Here's how the part is built. I have some questions about the finished solid (model axes, mm). Face numbers are marked on the shaded views. A direction names the side the tool comes from. Coordinates: 2 decimals unless noted, no trailing zeros. Write each loop counter-clockwise with the first axis right and the second up, starting at its lowest first coordinate (ties: lowest second). Pieces come first, ordered by that corner, then holes.
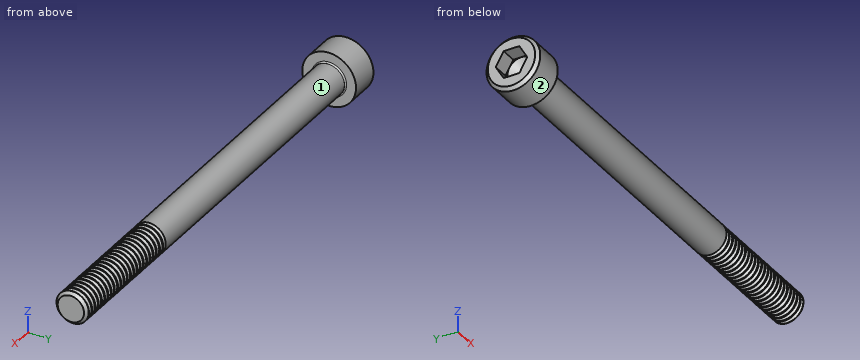
```python
from build123d import *

# Parameters (mm, degrees)
FILLET1_R       = 0.25
HEX_2_DEPTH     = 3
THDSCHPAT_COUNT = 24
THDSCHPAT_PITCH = 1


with BuildPart() as part:
    # BodySke → Base-Revolve (revolve)
    with BuildSketch(Plane.XY):
        Polygon((0, 0), (0, 4.4), (0.6, 5), (6, 5), (6, 3), (85.4455, 3), (86, 2.4455), (86, 0), align=None)
    revolve(axis=Axis((-31.75, 0, 0), (1, 0, 0)))

    # Fillet1
    fillet1_edges = [part.edges().sort_by_distance(p)[0] for p in [
        (6, -3, 0),
    ]]
    fillet(fillet1_edges, radius=FILLET1_R)

    # Sketch2 → Hex-PreBroach (revolve, cut)
    with BuildSketch(Plane.XY):
        Polygon((0, 2.542), (3, 2.542), (4.467624384, 0), (0, 0), align=None)
    revolve(axis=Axis((0, 0, 0), (1, 0, 0)), mode=Mode.SUBTRACT)

    # Sketch3 → Hex 2 (cut)
    with BuildSketch(Plane(origin=(0, 0, 0), x_dir=(0, 0.5, 0.866025404), z_dir=(-1, 0, 0))):
        Polygon((1.467624384, 2.542), (-1.467624384, 2.542), (-2.935248769, 0), (-1.467624384, -2.542), (1.467624384, -2.542), (2.935248769, 0), align=None)
    extrude(amount=-HEX_2_DEPTH, mode=Mode.SUBTRACT)

    # ThdSchSke → ThreadSchematic (revolve, cut)
    with BuildSketch(Plane.XY):
        Polygon((62, -2.4455), (61.61173492, -3), (61.61173492, -3.75), (62.38826508, -3.75), (62.38826508, -3), align=None)
    threadschematic = revolve(axis=Axis((-3.175, 0, 0), (1, 0, 0)), mode=Mode.SUBTRACT)

    # ThdSchPat: ThreadSchematic ×24
    with Locations(*[(i * THDSCHPAT_PITCH, 0, 0) for i in range(1, THDSCHPAT_COUNT)]):
        add(threadschematic, mode=Mode.SUBTRACT)


solid = part.part
```
1) Will these pins go through, and if not, where does the flat tip stop? pin 1 (5 mm diameter, centred on x = 43.5, y = 4, fed in from -Z); pin 2 (2 mm diameter, centred on x = 24, y = 0, fed in from +Z); pin 3 (1.5 mm diameter, centred on x = 74, z = -2.5, fed in from -Y).
Values follow:
pin 1: stops at z = -2.6
pin 2: stops at z = 3
pin 3: stops at y = -2.36
2) Imagine slicing it at A-A on x = 24.5. Please give me the cut outline in (y, z).
Values follow:
outline: circle Ø6 at (0, 0)
3) I need wall thicknesses on probe 1 along Z at (x, y) = (26.5, -0.25); probe 2 along Y at (x, z) = (5, -4); probe 3 along X at (y, z) = (1, 3.5). Which ranges of each line are inside material? Lowest first, please.
Values follow:
probe 1: z = -2.99 to 2.99
probe 2: y = -3 to 3
probe 3: x = 0 to 6
4) On a 3-axis mill with a long thin cutter (end or side, diameter ignored), from which of +Z, -Z, +X, -X, +Y, -Y can I reach the whole of each face in a straight line? I mean the marked faces 1 and 2. Say none if no direction works.
Values follow:
face 1: +X
face 2: +X, -X
